```python
from build123d import *

# Parameters (mm, degrees)
SKETCH1_W                                    = 70
SKETCH1_H                                    = 25
SKETCH1_R                                    = 1.35
BOSS_EXTRUDE1_DEPTH                          = 6
CHAMFER1_SIZE                                = 0.5
FILLET1_R                                    = 10
CHAMFER2_SIZE                                = 0.5
CSK_FOR_M3_COUNTERSUNK_FLAT_HEAD_SCR_2_COUNT = 2
CSK_FOR_M3_COUNTERSUNK_FLAT_HEAD_SCR_2_PITCH = 32


with BuildPart() as part:
    # Sketch1 → Boss-Extrude1 (new body)
    with BuildSketch(Plane.XY):
        Rectangle(SKETCH1_W, SKETCH1_H)
        with Locations((-27, 0)):
            Circle(SKETCH1_R, mode=Mode.SUBTRACT)
        with Locations((27, 0)):
            Circle(SKETCH1_R, mode=Mode.SUBTRACT)
        with Locations((-16, 0)):
            Circle(SKETCH1_R, mode=Mode.SUBTRACT)
        with Locations((16, 0)):
            Circle(SKETCH1_R, mode=Mode.SUBTRACT)
    extrude(amount=BOSS_EXTRUDE1_DEPTH)

    # Chamfer1
    chamfer1_edges = [part.edges().sort_by_distance(p)[0] for p in [
        (-28.35, 0, 0),
        (-28.35, 0, 6),
        (25.65, 0, 0),
        (25.65, 0, 6),
    ]]
    chamfer(chamfer1_edges, length=CHAMFER1_SIZE)

    # Fillet1
    fillet1_edges = [part.edges().sort_by_distance(p)[0] for p in [
        (35, -12.5, 3),
        (-35, -12.5, 3),
        (-35, 12.5, 3),
        (35, 12.5, 3),
    ]]
    fillet(fillet1_edges, radius=FILLET1_R)

    # Chamfer2
    chamfer2_edges = [part.edges().sort_by_distance(p)[0] for p in [
        (-35, 0, 0),
        (-35, 0, 6),
        (35, 0, 0),
        (0, -12.5, 0),
        (0, 12.5, 0),
        (32.071067812, -9.571067812, 0),
        (-32.071067812, -9.571067812, 0),
        (32.071067812, 9.571067812, 0),
        (-32.071067812, 9.571067812, 0),
        (0, 12.5, 6),
        (35, 0, 6),
        (0, -12.5, 6),
        (32.071067812, -9.571067812, 6),
        (-32.071067812, -9.571067812, 6),
        (32.071067812, 9.571067812, 6),
        (-32.071067812, 9.571067812, 6),
    ]]
    chamfer(chamfer2_edges, length=CHAMFER2_SIZE)

    # Sketch3 → CSK for M3 Countersunk Flat Head Screw1 (revolve, cut)
    with BuildSketch(Plane.YZ.offset(-16)):
        Polygon((0, 0), (0, 6), (1.825, 6), (1.8, 5.975), (1.8, 2.35), (4.15, 0), align=None)
    csk_for_m3_countersunk_flat_head_screw1 = revolve(axis=Axis((-16, 0, -6.35), (0, 0, 1)), mode=Mode.SUBTRACT)

    # CSK for M3 Countersunk Flat Head Scr 2: CSK for M3 Countersunk Flat Head Screw1 ×2
    with Locations(*[(i * CSK_FOR_M3_COUNTERSUNK_FLAT_HEAD_SCR_2_PITCH, 0, 0) for i in range(1, CSK_FOR_M3_COUNTERSUNK_FLAT_HEAD_SCR_2_COUNT)]):
        add(csk_for_m3_countersunk_flat_head_screw1, mode=Mode.SUBTRACT)


solid = part.part
```
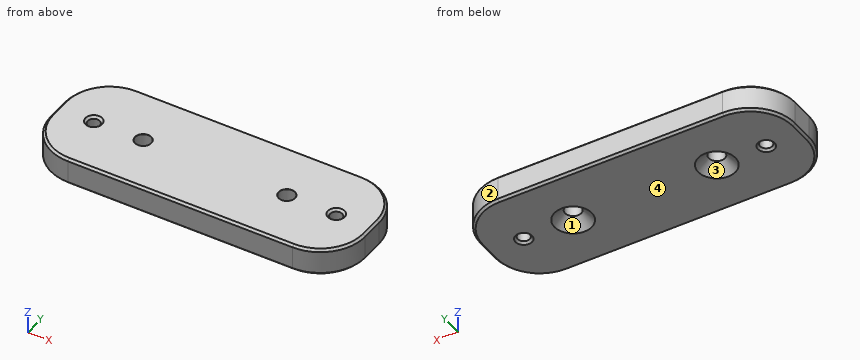
Model file for the job. Use its own axes, mm. Face numbers are marked on the shaded views. Give positions to 0.01 mm unless a question says otherwise; leave off trailing zeros. Loops run counter-clockwise (first coordinate to the right, second up) from the corner with the lowest first, then second, coordinate; pieces in that order, holes last. Notation, with made-up numbers: (-38.75, 65.25) -> (-0.75, 65.25) arc R21 cw to (-0.75, 96.25) -> close; hole circle Ø6 at (76.5, 78.25). An arc over 180 degrees is marked (long way). Use CSV: the item, a comma, the result in double quotes. Start each with the question number.
1) Slice it at A-A on z = 3.25. Give the cut face in (x, y), plus the area to 3 significant figures.
2) Wall check: line 1 (X direction, y = -1, z = 5); line 2 (Y direction, x = 16, z = 5.2); line 3 (X direction, y = -1.5, z = 1.75). Give the ranges that are in metal, low to high.
3) Flat gauge pins, fed straight in: pin 1 Ø1.5 at (y, z) = (4.5, 4) entering from -X; pin 2 Ø4.5 at (x, y) = (-16, 0) entering from -Z; pin 3 Ø3.5 at (x, y) = (-27, 0) entering from +Z. Where does each tip first touch, or does it go through?
4) Mould opens along X. For the marked faces 1, 2, 3 and 4 say: released by +X, released by -X, zero draft, split by the parting line, or undercut.
5) Slice it at B-B on x = 16. Give the cut face in (y, z) (3 decimals), plus the area to 3 significant figures.
Computed values:
1,outline,"(-35, -2.5) arc R10 ccw to (-25, -12.5) -> (25, -12.5) arc R10 ccw to (35, -2.5) -> (35, 2.5) arc R10 ccw to (25, 12.5) -> (-25, 12.5) arc R10 ccw to (-35, 2.5) -> close; hole circle Ø2.7 at (-27, 0); hole circle Ø3.6 at (-16, 0); hole circle Ø3.6 at (16, 0); hole circle Ø2.7 at (27, 0)"
1,area,"1,630 mm^2"
2,line 1,"x = -35 to -27.91, -26.09 to -17.5, -14.5 to 14.5, 17.5 to 26.09, 27.91 to 35"
2,line 2,"y = -12.5 to -1.8, 1.8 to 12.5"
2,line 3,"x = -35 to -17.87, -14.13 to 14.13, 17.87 to 35"
3,pin 1,"stops at x = -34.92"
3,pin 2,"stops at z = 1.9"
3,pin 3,"stops at z = 5.9"
4,face 1,"undercut"
4,face 2,"released by +X"
4,face 3,"undercut"
4,face 4,"zero draft"
5,outline,"(-12.5, 0.5) -> (-12, 0) -> (-4.15, 0) -> (-1.8, 2.35) -> (-1.8, 5.975) -> (-1.825, 6) -> (-12, 6) -> (-12.5, 5.5) -> close; (1.8, 2.35) -> (4.15, 0) -> (12, 0) -> (12.5, 0.5) -> (12.5, 5.5) -> (12, 6) -> (1.825, 6) -> (1.8, 5.975) -> close"
5,area,"122 mm^2"
